For this review, take the finished solid that the model builds, in its own axes (mm). A direction names the side the tool comes from. Coordinates: 2 decimals unless noted, no trailing zeros. Write each loop counter-clockwise with the first axis right and the second up, starting at its lowest first coordinate (ties: lowest second). Pieces come first, ordered by that corner, then holes. Notation, with made-up numbers: (-36.5, 19) -> (-11.5, 19) arc R22 cw to (-11.5, 57) -> close; hole circle Ø10 at (53, -14.5). An arc over 180 degrees is marked (long way). One line per item, written item: value. Start each with the question number.
1) Machinability: for faces 1 (the flat face through (3, -9, 3)), 2 (the flat face through (3, 0, 4)), 3 (the flat face through (1, 3.75, 1)), 4 (the flat face through (6, 10.75, 2)), which of the approach directions +Z, -Z, +X, -X, +Y, -Y give a long, thin tool a straight path to every point of the face, cutting with its end or side? Answer none if there is none.
2) For pin 1 Ø2 at (x, z) = (1.5, 3) entering from +Y; pin 2 Ø2.5 at (y, z) = (8, 3) entering from -X; pin 3 Ø2 at (x, z) = (1.5, 1.5) entering from -Y; pin 4 Ø3 at (y, z) = (0, 3) entering from -X, all flat-tipped, find the tip position at first contact; note any pin that passes through.
3) Add section B-B (z = 1.15). State the section outline as (x, y) points, and give its area (3 significant figures).
4) Add section D-D (x = 8.75). State the section outline as (y, z) points.
5) Mouldability with a two-part tool opening along X and no side actions: class faces 5 (the flat face through (1, -3.75, 1)), 6 (the flat face through (3, 9, 3)), 7 (the cylindrical face through (5.01, 4.76, 2.46)) as released by +X, released by -X, zero draft, split by the parting line, or undercut.
6) Add section C-C (y = -4.8). State the section outline as (x, z) points.
7) Add section A-A (x = 6). State the section outline as (y, z) points, and give its area (3 significant figures).
8) For probe 1 along Y at (x, z) = (6, 2.7); probe 2 along Z at (x, y) = (7.15, -7.75); probe 3 along Y at (x, z) = (5.75, 0.5), list the stretches that pass through material, from the lowest coordinate up. Write a range as from..to.
Autodesk Inventor part; units mm, degrees
ref_plane "YZ Plane" through (0, 0, 0) normal (1, 0, 0) x (0, 1, 0)
ref_plane "XZ Plane" through (0, 0, 0) normal (0, 1, 0) x (-1, 0, 0)
ref_plane "XY Plane" through (0, 0, 0) normal (0, 0, 1) x (1, 0, 0)
sketch "スケッチ1" plane through (0, 0, 0) normal (0, 0, 1) x (1, 0, 0)
  line L0 (0, -3.75) -> (0, 3.75)
  line L1 (0, -3.75) -> (3, -3.75)
  line L2 (3, -5.85) -> (3, -10.75)
  line L3 (3, -10.75) -> (9, -10.75)
  line L4 (9, -10.75) -> (9, 10.75)
  line L5 (0, 0) -> (9, 0) construction
  arc A0 (3, -5.85) -> (3, -3.75) centre (3, -4.8) ccw
  line L6 (3, -7.75) -> (9, -7.75) construction
  line L7 (3, -9.25) -> (9, -9.25) construction
  line L8 (3, -6.25) -> (9, -6.25) construction
  line L9 (0, 3.75) -> (3, 3.75)
  line L10 (3, 5.85) -> (3, 10.75)
  line L11 (3, 10.75) -> (9, 10.75)
  arc A1 (3, 3.75) -> (3, 5.85) centre (3, 4.8) ccw
  line L12 (3, 7.75) -> (9, 7.75) construction
  line L13 (3, 9.25) -> (9, 9.25) construction
  line L14 (3, 6.25) -> (9, 6.25) construction
  circle A2 centre (6, -4) radius 1.25
  circle A3 centre (6, 4) radius 1.25
  line L15 (6, -10.75) -> (6, 10.75) construction
  line L16 (3, 3.75) -> (3, -3.75)
  dimension "d0" = 3
  dimension "d1" = 6
  dimension "d2" = 1.05
  dimension "d3" = 7.5
  dimension "d4" = 21.5
  dimension "d5" = 3
  dimension "d6" = 15.5
  dimension "d7" = 2.5
  dimension "d9" = 8
extrude "押し出し1" add sketch "スケッチ1" along normal blind 5 contours L16 A1 L10 L11 L4 L3 L2 A0
extrude "押し出し2" add sketch "スケッチ1" along normal blind 2.5 contours L0 L9 L16 L1
sketch "スケッチ2" plane through (9, -10.75, 0) normal (1, 0, 0) x (0, 0, -1)
  line L0 (0, 10.75) -> (-5, 10.75) construction
  line L1 (-5, 0) -> (-5, 21.5)
  line L2 (0, 0) -> (-5, 0)
  line L3 (0, 21.5) -> (-5, 21.5)
  line L4 (-2, 0) -> (-2, 21.5) construction
  point P0 (-2, 3)
  point P1 (-2, 18.5)
  dimension "d13" = 15.5
  dimension "d23" = 3
hole "穴1" at (9, -7.75, 2) at (9, 7.75, 2) direction (-1, 0, 0) diameter 2.459 depth 6
properties part number "Foot_root_block" material "アルミニウム 2014-T4"
Numbers:
1. face 1: +Z, -Z, -X, -Y
1. face 2: +Z, -X, +Y, -Y
1. face 3: +Z, -Z, -X, +Y
1. face 4: +Z, -Z, +X, -X, +Y
2. pin 1: y = 3.75
2. pin 2: x = 3
2. pin 3: y = -3.75
2. pin 4: x = 0
3. outline: (0, -3.75) -> (3, -3.75) arc R1.05 cw to (3, -5.85) -> (3, -6.86) -> (9, -6.86) -> (9, 6.86) -> (3, 6.86) -> (3, 5.85) arc R1.05 cw to (3, 3.75) -> (0, 3.75) -> close; (3, -10.75) -> (9, -10.75) -> (9, -8.64) -> (3, -8.64) -> close; (3, 8.64) -> (9, 8.64) -> (9, 10.75) -> (3, 10.75) -> close; hole circle Ø2.5 at (6, -4); hole circle Ø2.5 at (6, 4)
3. area: 117 mm²
4. outline: (-10.75, 0) -> (10.75, 0) -> (10.75, 5) -> (-10.75, 5) -> close; hole circle Ø2.46 at (-7.75, 2); hole circle Ø2.46 at (7.75, 2)
5. face 5: zero draft
5. face 6: released by -X
5. face 7: undercut
6. outline: (4.05, 0) -> (5.04, 0) -> (5.04, 5) -> (4.05, 5) -> close; (6.96, 0) -> (9, 0) -> (9, 5) -> (6.96, 5) -> close
7. outline: (-10.75, 0) -> (-5.25, 0) -> (-5.25, 5) -> (-10.75, 5) -> close; (-2.75, 0) -> (2.75, 0) -> (2.75, 5) -> (-2.75, 5) -> close; (5.25, 0) -> (10.75, 0) -> (10.75, 5) -> (5.25, 5) -> close; hole circle Ø2.46 at (-7.75, 2); hole circle Ø2.46 at (7.75, 2)
7. area: 73.0 mm²
8. probe 1: -10.75..-8.76, -6.74..-5.25, -2.75..2.75, 5.25..6.74, 8.76..10.75
8. probe 2: 0..0.77, 3.23..5
8. probe 3: -10.75..-5.22, -2.78..2.78, 5.22..10.75
